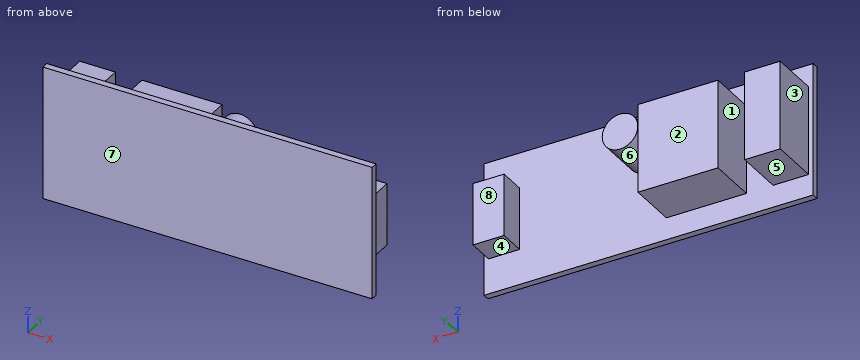
Autodesk Inventor part; units mm, degrees
ref_plane "YZ Plane" through (0, 0, 0) normal (1, 0, 0) x (0, 1, 0)
ref_plane "XZ Plane" through (0, 0, 0) normal (0, 1, 0) x (-1, 0, 0)
ref_plane "XY Plane" through (0, 0, 0) normal (0, 0, 1) x (1, 0, 0)
sketch "Sketch1" plane through (0, 0, 0) normal (0, 1, 0) x (-1, 0, 0)
  line L0 (0, 0) -> (-74, 0)
  line L1 (-74, 0) -> (-74, -30)
  line L2 (-74, -30) -> (0, -30)
  line L3 (0, -30) -> (0, 0)
  dimension "d0" = 74
  dimension "d1" = 30
extrude "Extrusion1" add sketch "Sketch1" along normal blind 1.5
sketch "Sketch2" plane through (0, 1.5, 0) normal (0, 1, 0) x (1, 0, 0)
  line L0 (0, 0) -> (74, 0) construction
  line L1 (0, 0) -> (0, 5) construction
  line L2 (0, 30) -> (0, 0) construction
  line L3 (0, 30) -> (0, 25) construction
  line L4 (0, 25) -> (42, 25)
  line L5 (42, 25) -> (42, 5)
  line L6 (42, 5) -> (0, 5)
  line L7 (0, 5) -> (0, 25)
  dimension "d4" = 5
  dimension "d5" = 5
  dimension "d6" = 42
extrude "Extrusion2" add sketch "Sketch2" along normal blind 11
sketch "Sketch3" plane through (0, 1.5, 0) normal (0, 1, 0) x (1, 0, 0)
  line L0 (74, 30) -> (0, 30) construction
  line L1 (74, 30) -> (74, 22) construction
  line L2 (74, 0) -> (74, 30) construction
  line L3 (0, 0) -> (74, 0) construction
  line L4 (74, 0) -> (74, 8) construction
  line L5 (74, 22) -> (66, 22)
  line L6 (66, 22) -> (66, 8)
  line L7 (66, 8) -> (74, 8)
  line L8 (74, 8) -> (74, 22)
  dimension "d9" = 8
  dimension "d10" = 8
  dimension "d11" = 8
extrude "Extrusion3" add sketch "Sketch3" along normal blind 6
sketch "Sketch4" plane through (0, 12.5, 0) normal (0, 1, 0) x (1, 0, 0)
  line L0 (0, 25) -> (42, 25)
  line L1 (42, 5) -> (0, 5)
  line L2 (0, 25) -> (9, 25)
  line L3 (9, 25) -> (9, 5)
  line L4 (9, 5) -> (0, 5)
  line L5 (0, 5) -> (0, 25)
  line L6 (0, 25) -> (32, 25)
  line L7 (32, 25) -> (32, 5)
  line L8 (32, 5) -> (0, 5)
  line L9 (0, 5) -> (0, 25)
  line L10 (32, 25) -> (15, 25)
  line L11 (15, 25) -> (15, 5)
  line L12 (15, 5) -> (32, 5)
  line L13 (32, 5) -> (32, 25)
  point P0 (0, 0)
  dimension "d14" = 9
  dimension "d15" = 32
  dimension "d16" = 17
extrude "Extrusion4" cut sketch "Sketch4" against normal up to surface (11 mm away) contours L0 L11 L1 L3
sketch "Sketch5" plane through (0, 12.5, 0) normal (0, 1, 0) x (1, 0, 0)
  line L0 (15, 5) -> (42, 5)
  line L1 (15, 25) -> (33, 25)
  line L2 (33, 25) -> (33, 5)
  line L3 (33, 5) -> (15, 5)
  line L4 (15, 5) -> (15, 25)
  line L5 (42, 25) -> (33, 25)
  line L6 (33, 25) -> (33, 5)
  line L7 (33, 5) -> (42, 5)
  line L8 (42, 5) -> (42, 25)
  point P0 (0, 0)
  dimension "d19" = 18
extrude "Extrusion5" cut sketch "Sketch5" against normal up to surface (11 mm away) contours L2 L5 L8 L0
sketch "Sketch6" plane through (0, 1.5, 0) normal (0, 1, 0) x (1, 0, 0)
  line L0 (0, 25) -> (9, 25) construction
  line L1 (0, 25) -> (42, 25) construction
  line L2 (42, 25) -> (42, 5) construction
  line L3 (42, 5) -> (0, 5) construction
  line L4 (0, 5) -> (0, 25) construction
  circle A0 centre (37.6164, 9.2055) radius 4
  point P0 (0, 0)
  dimension "d22" = 42
  dimension "d23" = 20
  dimension "d24" = 8
extrude "Extrusion6" add sketch "Sketch6" along normal blind 10
sketch "Sketch7" plane through (74, 0, 0) normal (1, 0, 0) x (0, 0, -1)
  point P0 (0, 0)
sketch "Sketch8" plane through (0, 0, -30) normal (-1, 0, 0) x (0, 0, 1)
  line L0 (25, 1.5) -> (25, 12.5)
  line L1 (25, 1.5) -> (5, 1.5)
  line L2 (25, 12.5) -> (5, 12.5)
  line L3 (5, 12.5) -> (5, 1.5)
  line L4 (5, 1.5) -> (25, 1.5)
  line L5 (25, 1.5) -> (25, 12.5)
  point P0 (30, 0)
extrude "Extrusion7" cut sketch "Sketch8" against normal blind 1
sketch "Sketch9" plane through (74, 0, 0) normal (1, 0, 0) x (0, 0, -1)
  line L0 (8, 1.5) -> (8, 7.5)
  line L1 (22, 1.5) -> (22, 7.5)
  line L2 (8, 7.5) -> (22, 7.5)
  line L3 (22, 7.5) -> (22, 1.5)
  line L4 (22, 1.5) -> (8, 1.5)
  line L5 (8, 1.5) -> (8, 7.5)
  point P0 (0, 0)
extrude "Extrusion8" cut sketch "Sketch9" against normal blind 1
properties part number "PZEM-00ET"
Model file for the job. Use its own axes, mm. Face numbers are marked on the shaded views. A direction names the side the tool comes from. Coordinates: 2 decimals unless noted, no trailing zeros. Order: outer loops, then holes, each group sorted by start corner. A loop starts at its lowest first (then second) coordinate and runs counter-clockwise, first axis right, second up. Notation, with made-up numbers: (-14, -37) -> (-2, -37) arc R31 cw to (-2, -6) -> close; hole circle Ø9 at (50, 35.25). An arc over 180 degrees is marked (long way). Answer as a JSON object with one key per item and string values. Group by question number.
1) Cut at D-D, the plane x = 47.5. Write the cut outline in (y, z).
2) Which spindle directions (+Z, -Z, +X, -X, +Y, -Y) get a long thin tool onto all of the face, cutting with end or side? Do the marked faces 4, 5, 6, 7 and 8. Say none if no direction does.
3) Drill centre lines: L1, parallel to X at y = 4.75, z = -9.25; L2, parallel to X at y = 2, z = -18; L3, parallel to X at y = 9.5, z = -23.75. Where is each one in solid material? Low to high.
4) Flat gauge pins, fed straight in: pin 1 (3 mm diameter, centred on y = 4, z = -5.5, fed in from -X); pin 2 (1 mm diameter, centred on x = 32, z = -18.5, fed in from -Y); pin 3 (3.5 mm diameter, centred on y = 5.5, z = -11.5, fed in from +X); pin 4 (5.5 mm diameter, centred on x = 27, y = 6.5, fed in from +Z). Where does each tip first touch, or does it go through?
5) Cut at C-C, the plane x = 30.5. Write the cut outline in (y, z).
6) Pull direction X, two halves, no side cores. Call the marked faces 1, 2 and 3: +X half, -X half, draft (parallel to the pull), parting line (faces both ways), or undercut.
7) Cut at A-A, the plane y = 6.75. Write the cut outline in (x, z), then the cut area to 3 significant figures.
8) Cut at B-B, the plane z = -20. Write the cut outline in (x, y).
Check values:
{
 "1": {"outline": "(0, -30) -> (1.5, -30) -> (1.5, 0) -> (0, 0) -> close"},
 "2": {"face 4": "-Z, +X, +Y", "face 5": "-Z, +X, -X, +Y", "face 6": "+Y", "face 7": "+Z, -Z, +X, -X, -Y", "face 8": "+Z, -Z, +X, +Y"},
 "3": {"L1": "x = 1 to 9, 15 to 33, 33.62 to 41.62, 66 to 73", "L2": "x = 1 to 9, 15 to 33, 66 to 73", "L3": "x = 1 to 9, 15 to 33"},
 "4": {"pin 1": "stops at x = 1", "pin 2": "stops at y = 0", "pin 3": "stops at x = 73", "pin 4": "stops at z = -5"},
 "5": {"outline": "(0, -30) -> (1.5, -30) -> (1.5, -25) -> (12.5, -25) -> (12.5, -5) -> (1.5, -5) -> (1.5, 0) -> (0, 0) -> close"},
 "6": {"face 1": "undercut", "face 2": "draft", "face 3": "-X half"},
 "7": {"outline": "(1, -25) -> (9, -25) -> (9, -5) -> (1, -5) -> close; (15, -25) -> (33, -25) -> (33, -5) -> (15, -5) -> close; circle Ø8 at (37.62, -9.21); (66, -22) -> (73, -22) -> (73, -8) -> (66, -8) -> close", "area": "668 mm²"},
 "8": {"outline": "(0, 0) -> (74, 0) -> (74, 1.5) -> (73, 1.5) -> (73, 7.5) -> (66, 7.5) -> (66, 1.5) -> (33, 1.5) -> (33, 12.5) -> (15, 12.5) -> (15, 1.5) -> (9, 1.5) -> (9, 12.5) -> (1, 12.5) -> (1, 1.5) -> (0, 1.5) -> close"}
}
